Autodesk Inventor part; units mm, degrees
ref_plane "工作平面1" through (10, 0, 0) normal (1, 0, 0) x (0, 1, 0)
ref_plane "XZ Plane" through (0, 0, 0) normal (0, 1, 0) x (-1, 0, 0)
ref_plane "XY Plane" through (0, 0, 0) normal (0, 0, 1) x (1, 0, 0)
sketch "草图1" plane through (0, 0, 0) normal (1, 0, 0) x (0, 1, 0)
  line L0 (0, 0) -> (20, 0)
  line L1 (20, 0) -> (20, -40)
  line L2 (20, -40) -> (0, -40)
  line L3 (0, -40) -> (0, 0)
  dimension "d0" = 20
  dimension "d1" = 40
ref_plane "工作平面1" through (10, 0, 0) normal (1, 0, 0) x (0, 1, 0)
sketch "草图2" plane through (10, 0, 0) normal (1, 0, 0) x (0, 1, 0)
  line L0 (0, 0) -> (30, 0)
  line L1 (30, 0) -> (30, -30)
  line L2 (30, -30) -> (0, -30)
  line L3 (0, -30) -> (0, 0)
  dimension "d7" = 30
  dimension "d8" = 30
loft "放样1" add profiles "草图2", "草图1"
sketch "草图3" plane through (10, 0, 0) normal (1, 0, 0) x (0, 0, -1)
  line L0 (0, 0) -> (0, 30)
  line L1 (30, 0) -> (0, 0)
  point P0 (5.5, 10)
  point P1 (26.5, 10)
  dimension "d14" = 21
  dimension "d15" = 5.5
  dimension "d16" = 10
hole "孔1" at (10, 10, -5.5) at (10, 10, -26.5) direction (-1, 0, 0) diameter 3.1 end through all countersink diameter 6 countersink angle 90
sketch "草图5" plane through (0, 0, 0) normal (-1, 0, 0) x (0, 0, 1)
  line L0 (0, 0) -> (0, 20)
  point P0 (-15, 15)
  dimension "d26" = 15
  dimension "d27" = 15
hole "孔2" at (0, 15, -15) direction (1, 0, 0) diameter 3.1 end through all countersink diameter 6 countersink angle 90
sketch "草图6" plane through (10, 0, 0) normal (1, 0, 0) x (0, 0, -1)
  line L0 (0, 30) -> (30, 30)
  line L1 (10.95, 30) -> (19.05, 30)
  line L2 (19.05, 30) -> (19.05, 25)
  line L3 (19.05, 25) -> (10.95, 25)
  line L4 (10.95, 25) -> (10.95, 30)
  line L5 (30, 0) -> (0, 0)
  line L6 (10.95, 5) -> (19.05, 5)
  line L7 (19.05, 5) -> (19.05, 0)
  line L8 (19.05, 0) -> (10.95, 0)
  line L9 (10.95, 0) -> (10.95, 5)
  line L10 (0, 0) -> (0, 30)
  point P0 (15, 30)
  dimension "d35" = 8.1
  dimension "d36" = 5
  dimension "d37" = 15
extrude "拉伸1" add sketch "草图6" along normal blind 3
chamfer "倒角1" distance 2 angle 45 8 edges at (5, 25, 0) (5, 25, -35) (5, 0, -35) (0, 10, -40) (0, 0, -20) (5, 0, 0) (0, 20, -20) (0, 10, 0)
properties part number "电源支架"
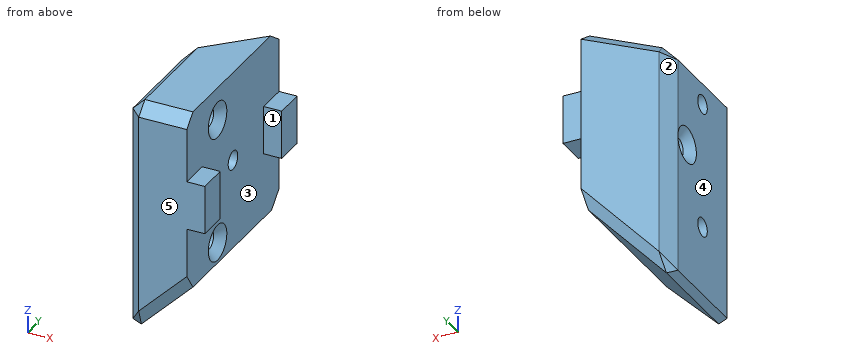
The model under review builds one solid part; all positions refer to its coordinate system, in mm. Face numbers are marked on the shaded views. A direction names the side the tool comes from. Give positions to 0.01 mm unless a question says otherwise; leave off trailing zeros. Write each loop counter-clockwise with the first axis right and the second up, starting at its lowest first coordinate (ties: lowest second). Pieces come first, ordered by that corner, then holes.
1. For P1, Ø3.5, axis at x = 11.5, y = 2, coming from the -Z side; P2, Ø0.9, axis at x = 12, y = 2.5, coming from the +Z side; P3, Ø4, axis at x = 5.5, z = -5, coming from the +Y side; P4, Ø2, axis at x = 3, z = -18, coming from the -Y side, all flat-tipped, find the tip position at first contact; note any pin that passes through.
2. Add section C-C, the plane x = 7. Count the separate pieces of the cut face and the enclosed holes in it, plus the area to 3 significant figures.
3. Draft analysis for pull direction Y (two halves, no side actions). For the marked faces 3, 4 and 5, state which applies: +Y half, -Y half, draft (parallel to the pull), parting line (faces both ways), or undercut.
4. Wall thickness on L1, parallel to Y at x = 5, z = -26.5; L2, parallel to Z at x = 6.25, y = 10; L3, parallel to X at y = 27, z = -19.5: over which ranges is each line inside the solid? List them lowest first.
5. Add section A-A, the plane x = 11. Write out the cut boundary in (y, z), plus the area to 3 significant figures.
6. Add section B-B, the plane x = 1. Write out the cut boundary in (y, z).
7. Tool access review of the marked faces 1 and 2: name each direction out of +Z, -Z, +X, -X, +Y, -Y from which nothing blocks a thin tool from reaching the whole face with its end or side.
Worked answers:
1. P1: stops at z = -30.25
1. P2: stops at z = -10.95
1. P3: stops at y = 27.5
1. P4: stops at y = 0
2. separate pieces: 1
2. enclosed holes: 3
2. area: 858 mm2
3. face 3: undercut
3. face 4: draft
3. face 5: -Y half
4. L1: y = 0 to 8.45, 11.55 to 25
4. L2: z = -33.75 to -28.05, -24.95 to -7.05, -3.95 to 0
4. L3: x = 7 to 10
5. outline: (0, -19.05) - (5, -19.05) - (5, -10.95) - (0, -10.95) - close; (25, -19.05) - (30, -19.05) - (30, -10.95) - (25, -10.95) - close
5. area: 81.0 mm2
6. outline: (1, -36.59) - (2, -38.41) - (18.68, -38.41) - (20.41, -36.68) - (20.41, -2) - (18.59, -1) - (2, -1) - (1, -2) - close; hole circle Ø3.1 at (10, -26.5); hole circle Ø3.1 at (10, -5.5); hole circle Ø4 at (15, -15)
7. face 1: +Z, -Z, +X
7. face 2: +Z, -Z, -X, +Y
